Could you check a few things on this model? Use its own coordinates, in mm. Round coordinates to 2 decimals unless told otherwise and drop trailing zeros. Loops run counter-clockwise (first coordinate to the right, second up) from the corner with the lowest first, then second, coordinate; pieces in that order, holes last.
from build123d import *

# Parameters (mm, degrees)
DODANIE_WYCI_GNI_CIE1_DEPTH       = 2
WYCI_GNI_CIE_CIENKA_CIANKA1_DEPTH = 10
SZKIC3_R                          = 2.5
WYTNIJ_WYCI_GNI_CIE1_DEPTH        = 10


with BuildPart() as part:
    # Szkic1 → Dodanie-wyciągnięcie1 (new body)
    with BuildSketch(Plane(origin=(184.050171811, 0, -211.725502995), x_dir=(-0.75470958, 0, -0.656059029), z_dir=(0.656059029, 0, -0.75470958))):
        with BuildLine():
            Line((-722.617736481, -314.120725024), (-723.785887875, -289.14803149))
            Line((-723.785887875, -289.14803149), (-703.807733048, -288.213510375))
            Line((-703.807733048, -288.213510375), (-702.74076796, -311.023047123))
            add(Edge.make_bspline(
                [(-722.617736481, -314.120725024), (-715.581558407, -312.012536185), (-708.710440218, -310.976356299), (-702.74076796, -311.023047123)],
                knots=[0.744519777, 0.744519777, 0.744519777, 0.744519777, 0.831521887, 0.831521887, 0.831521887, 0.831521887], degree=3, weights=[0.500240263, 0.497697377, 0.515339471, 0.553166544]))
        make_face()
    extrude(amount=DODANIE_WYCI_GNI_CIE1_DEPTH)

    # Szkic2 → Wyciągnięcie-cienka ścianka1 (add)
    with BuildSketch(Plane(origin=(185.362289869, 0, -213.234922155), x_dir=(-0.75470958, 0, -0.656059029), z_dir=(0.656059029, 0, -0.75470958))):
        Polygon((-723.785887875, -289.14803149), (-703.807733048, -288.213510375), (-703.714280936, -290.211325858), (-723.692435763, -291.145846973), align=None)
    extrude(amount=WYCI_GNI_CIE_CIENKA_CIANKA1_DEPTH)

    # Szkic3 → Wytnij-wyciągnięcie1 (cut)
    with BuildSketch(Plane(origin=(-9.063445171, -256.731823112, -7.878732686), x_dir=(-0.999377978, 0.035240125, 0.001338532), z_dir=(-0.035264602, -0.998907741, -0.030655051))):
        with Locations((-736.736241375, -260.210465694)):
            Circle(SZKIC3_R)
    extrude(amount=-WYTNIJ_WYCI_GNI_CIE1_DEPTH, mode=Mode.SUBTRACT)


solid = part.part
Item 1: If we section it at A-A, the plane z = 244.5: Please give me the cut outline in (x, y).
Results list:
outline: (719.89, -290.21) - (727.17, -290.47) - (727.17, -288.47) - (720.01, -288.21) - close
Item 2: If I drill on line 1 along Z through (x, y) = (729.5, -290); line 2 along Y through (x, z) = (735.25, 255.75); line 3 along Y through (x, z) = (723, 244.25), over which ranges is the centre line in solid material (lowest first)?
Results list:
line 1: z = 246.53 to 250.05, 252.45 to 262.43
line 2: y = -291.1 to -289.1
line 3: y = -290.31 to -288.31
Item 3: If we section it at B-B, the plane y = -305.25: Please give me the cut outline in (x, z).
Results list:
outline: (714.62, 249.49) - (715.93, 247.98) - (731.04, 261.12) - (729.73, 262.63) - close
Item 4: We'd pull the mould along X, two halves only. Please class faces 1 (the cylindrical face through (729.812, -289.778, 251.14)), 2 (the flat face through (722.246, -300.986, 256.121)), 3 (the flat face through (730.491, -289.659, 247.388)): released by +X, released by -X, zero draft, split by the parting line, or undercut.
Results list:
face 1: undercut
face 2: released by -X
face 3: released by +X
Item 5: Will these pins go through, and if not, where does the flat tip stop? pin 1 (1 mm diameter, centred on x = 727.5, z = 255, fed in from -Y); pin 2 (8 mm diameter, centred on y = -299, z = 260, fed in from -X); pin 3 (1 mm diameter, centred on x = 729.5, z = 256, fed in from +Y).
Results list:
pin 1: stops at y = -290.83
pin 2: stops at x = 722.11
pin 3: stops at y = -288.88
